```python
from build123d import *

# Parameters (mm, degrees)
BOSS_EXTRUDE1_DEPTH = 16.5735
SKETCH2_W           = 7.62
SKETCH2_H           = 7.62
SKETCH2_W_2         = 5.588
SKETCH2_H_2         = 5.588
BOSS_EXTRUDE2_DEPTH = 52.197


with BuildPart() as part:
    # Sketch1 → Boss-Extrude1 (new body, symmetric)
    with BuildSketch(Plane.XY):
        with BuildLine():
            Line((0, 0), (0, 19.177))
            Line((0, 19.177), (-10.795, 19.177))
            Line((-10.795, 19.177), (-10.795, 6.096))
            Line((-10.795, 6.096), (-24.892, 6.096))
            ThreePointArc((-24.892, 6.096), (-26.957458908, 6.951541092), (-27.813, 9.017))
            Line((-27.813, 9.017), (-29.083, 9.017))
            Line((-29.083, 9.017), (-29.083, 3.81))
            ThreePointArc((-29.083, 3.81), (-27.967076836, 1.115923164), (-25.273, 0))
            Line((-25.273, 0), (0, 0))
        make_face()
    extrude(amount=BOSS_EXTRUDE1_DEPTH, both=True)

    # Sketch2 → Boss-Extrude2 (add)
    with BuildSketch(Plane(origin=(0, 19.177, 0), x_dir=(1, 0, 0), z_dir=(0, 1, 0))):
        with Locations((-5.3975, 10.9855)):
            Rectangle(SKETCH2_W, SKETCH2_H)
        with Locations((-5.3975, 10.9855)):
            Rectangle(SKETCH2_W_2, SKETCH2_H_2, mode=Mode.SUBTRACT)
        with Locations((-5.3975, -10.9855)):
            Rectangle(SKETCH2_W, SKETCH2_H)
        with Locations((-5.3975, -10.9855)):
            Rectangle(SKETCH2_W_2, SKETCH2_H_2, mode=Mode.SUBTRACT)
    extrude(amount=BOSS_EXTRUDE2_DEPTH)


solid = part.part
```
Could you check a few things on this model? Use its own coordinates, in mm. A direction names the side the tool comes from. Coordinates: 2 decimals unless noted, no trailing zeros. Write each loop counter-clockwise with the first axis right and the second up, starting at its lowest first coordinate (ties: lowest second). Pieces come first, ordered by that corner, then holes. Notation, with made-up numbers: (69.5, 48) - (74.5, 48) arc R17 ccw to (74.5, 75) - close; hole circle Ø11 at (-13.5, 86). An arc over 180 degrees is marked (long way). Use a Markdown table: item, result.
Q1. Imagine slicing it at D-D (z = 10). List the corners of the cut face in (x, y) for me (1 decimal), and give its area (3 significant figures).
Geometry check:
| item | result |
|---|---|
| outline | (-29.1, 3.8) arc R3.8 ccw to (-25.3, 0) - (0, 0) - (0, 19.2) - (-1.6, 19.2) - (-1.6, 71.4) - (-2.6, 71.4) - (-2.6, 19.2) - (-8.2, 19.2) - (-8.2, 71.4) - (-9.2, 71.4) - (-9.2, 19.2) - (-10.8, 19.2) - (-10.8, 6.1) - (-24.9, 6.1) arc R2.9 cw to (-27.8, 9) - (-29.1, 9) - close |
| area | 427 mm2 |
Q2. I'm going to push flat-ended pins straight in: pin 1 Ø6 at (y, z) = (51.5, -12) entering from -X; pin 2 Ø8.5 at (y, z) = (58, -10.5) entering from +X; pin 3 Ø4 at (x, y) = (-3.5, 29) entering from +Z. Where does each tip first touch, or does it pass through?
Geometry check:
| item | result |
|---|---|
| pin 1 | stops at x = -9.21 |
| pin 2 | stops at x = -1.59 |
| pin 3 | stops at z = 14.8 |
Q3. Which directions (+Z, -Z, +X, -X, +Y, -Y) give clear straight access to the entire face, cutting with the end or side of a thin tool? Please do faces 4 (the flat face through (-1.588, 45, -11)), 5 (the flat face through (-5, 45, 8.192)), 6 (the flat face through (-10.795, 13, 0)).
Geometry check:
| item | result |
|---|---|
| face 4 | +Z, -Z, +X, +Y |
| face 5 | +Y |
| face 6 | +Z, -Z, +Y |
Q4. Imagine slicing it at B-B (z = 1). List the corners of the cut face in (x, y) for me (3 decimals).
Geometry check:
| item | result |
|---|---|
| outline | (-29.083, 3.81) arc R3.81 ccw to (-25.273, 0) - (0, 0) - (0, 19.177) - (-10.795, 19.177) - (-10.795, 6.096) - (-24.892, 6.096) arc R2.921 cw to (-27.813, 9.017) - (-29.083, 9.017) - close |
Q5. Imagine slicing it at A-A (y = 37). List the corners of the cut face in (x, z) for me, and give its area (3 significant figures).
Geometry check:
| item | result |
|---|---|
| outline | (-9.21, -14.8) - (-1.59, -14.8) - (-1.59, -7.18) - (-9.21, -7.18) - close; (-9.21, 7.18) - (-1.59, 7.18) - (-1.59, 14.8) - (-9.21, 14.8) - close; hole (-8.19, -13.78) - (-2.6, -13.78) - (-2.6, -8.19) - (-8.19, -8.19) - close; hole (-8.19, 8.19) - (-2.6, 8.19) - (-2.6, 13.78) - (-8.19, 13.78) - close |
| area | 53.7 mm2 |
Q6. Please list where these lines run through material, in increasing order: L1, parallel to Z at x = -6.5, y = 53; L2, parallel to X at y = 64.5, z = -10; L3, parallel to Y at x = -24.25, z = -13.
Geometry check:
| item | result |
|---|---|
| L1 | z = -14.8 to -13.78, -8.19 to -7.18, 7.18 to 8.19, 13.78 to 14.8 |
| L2 | x = -9.21 to -8.19, -2.6 to -1.59 |
| L3 | y = 0 to 6.1 |
Q7. Imagine slicing it at C-C (x = -13.75). List the corners of the cut face in (y, z) for me.
Geometry check:
| item | result |
|---|---|
| outline | (0, -16.57) - (6.1, -16.57) - (6.1, 16.57) - (0, 16.57) - close |
Q8. Thinking about a two-plate mould opening in Z: for faces 1 (the flat face through (-5, 45, -14.796)), 2 (the flat face through (-5, 45, -7.176)), 3 (the flat face through (-13, 0, 0)), which applies, +Z half, -Z half, draft (parallel to the pull), parting line (faces both ways), or undercut?
Geometry check:
| item | result |
|---|---|
| face 1 | -Z half |
| face 2 | undercut |
| face 3 | draft |
